from build123d import *

# Parameters (mm, degrees)
BOSS_EXTRUDE1_DEPTH          = 25.4
FILLET1_R                    = 0.79375
M2_5_CLEARANCE_HOLE1_D       = 2.9
M2_5X0_45_TAPPED_HOLE1_D     = 2.05
M2_5X0_45_TAPPED_HOLE1_DEPTH = 3.956117865
M2_5X0_45_TAPPED_HOLE1_TIP   = 0.615882135
F_4_CLEARANCE_HOLE1_D        = 3.2639


with BuildPart() as part:
    # Sketch1 → Boss-Extrude1 (new body)
    with BuildSketch(Plane.XY):
        with BuildLine():
            Line((-4.7625, 2.38125), (4.7625, 2.38125))
            Line((4.7625, 2.38125), (4.7625, 23.01875))
            Line((4.7625, 23.01875), (9.525, 23.01875))
            Line((9.525, 23.01875), (9.525, 5.55625))
            ThreePointArc((9.525, 5.55625), (10.45493597, 3.31118597), (12.7, 2.38125))
            Line((12.7, 2.38125), (22.225, 2.38125))
            Line((22.225, 2.38125), (22.225, -2.38125))
            Line((22.225, -2.38125), (-22.225, -2.38125))
            Line((-22.225, -2.38125), (-22.225, 2.38125))
            Line((-22.225, 2.38125), (-12.7, 2.38125))
            ThreePointArc((-12.7, 2.38125), (-10.45493597, 3.31118597), (-9.525, 5.55625))
            Line((-9.525, 5.55625), (-9.525, 23.01875))
            Line((-9.525, 23.01875), (-4.7625, 23.01875))
            Line((-4.7625, 23.01875), (-4.7625, 2.38125))
        make_face()
    extrude(amount=BOSS_EXTRUDE1_DEPTH)

    # Fillet1
    fillet1_edges = [part.edges().sort_by_distance(p)[0] for p in [
        (-4.7625, 2.38125, 12.7),
        (4.7625, 2.38125, 12.7),
    ]]
    fillet(fillet1_edges, radius=FILLET1_R)

    # M2.5 Clearance Hole1 (through all)
    with Locations(Plane(origin=(0, 2.38125, 0), x_dir=(1, 0, 0), z_dir=(0, 1, 0))):
        with Locations((17.5006, -4.70027), (17.5006, -20.69973), (-17.5006, -20.69973), (-17.5006, -4.70027)):
            Hole(M2_5_CLEARANCE_HOLE1_D / 2)

    # M2.5x0.45 Tapped Hole1
    with Locations(Plane(origin=(0, -2.38125, 0), x_dir=(-1, 0, 0), z_dir=(0, -1, 0))):
        with Locations((-7.78002, -4.70027), (7.78002, -4.70027), (7.78002, -20.69973), (-7.78002, -20.69973)):
            Hole(M2_5X0_45_TAPPED_HOLE1_D / 2, depth=M2_5X0_45_TAPPED_HOLE1_DEPTH)
            with Locations((0, 0, -(M2_5X0_45_TAPPED_HOLE1_DEPTH + M2_5X0_45_TAPPED_HOLE1_TIP / 2))):  # 118° drill point
                Cone(0, M2_5X0_45_TAPPED_HOLE1_D / 2, M2_5X0_45_TAPPED_HOLE1_TIP, mode=Mode.SUBTRACT)

    # #4 Clearance Hole1 (through all)
    with Locations(Plane.ZY.offset(9.525)):
        with Locations((6.35, 18.25625), (19.05, 18.25625), (19.05, 8.73125), (6.35, 8.73125), (12.7, 13.49375)):
            Hole(F_4_CLEARANCE_HOLE1_D / 2)


solid = part.part
Can you work these out from the model? Positions are in its coordinate system, mm. A direction names the side the tool comes from. Round coordinates to 2 decimals unless told otherwise and drop trailing zeros. Loops run counter-clockwise (first coordinate to the right, second up) from the corner with the lowest first, then second, coordinate; pieces in that order, holes last. Notation, with made-up numbers: (85, 72) - (101, 72) arc R15 cw to (101, 99) - close; hole circle Ø11 at (73.5, 18). An arc over 180 degrees is marked (long way). Use CSV: the item, a comma, the result in double quotes. Start each with the question number.
1) For pin 1 Ø3 at (x, z) = (-18.5, 12.5) entering from +Y; pin 2 Ø6 at (y, z) = (14, 15) entering from +X (3 decimals); pin 3 Ø5 at (y, z) = (10.5, 17) entering from -X (3 decimals), each with a flat end and sliding along its axis, tell me the tip position at first contact or that it passes through.
2) If we section it at A-A on z = 12.7: Count the separate pieces of the cut face and the enclosed holes in it, plus the area to 3 significant figures.
3) Please list where these lines run through material, in increasing order: probe 1 along Y at (x, z) = (-7.5, 6.35); probe 2 along X at (y, z) = (20, 19.75) (1 decimal); probe 3 along Z at (x, y) = (-6.5, 18.5). Write a range as [from, to].
4) We'd pull the mould along X, two halves only. Please class faces 1 (the cylindrical face through (8.331, -0.375, 3.836)), 2 (the flat face through (9.525, 16, 13)), 3 (the flat face through (-9.525, 16, 13)), 4 (the cylindrical face through (7.18, 8.8, 20.68)): released by +X, released by -X, zero draft, split by the parting line, or undercut.
5) For faces 5 (the flat face through (0, 2.381, 13)), 6 (the cylindrical face through (8.331, -0.375, 19.835)), 7 (the flat face through (-2, 2, 25.4)), which set-ups out of +Z, -Z, +X, -X, +Y, -Y let a thin tool reach every point of the face, with its end or its side?
6) If we section it at D-D on x = -14: Write out the boundary of the cut face in (y, z), plus the area to 3 significant figures.
7) If we section it at B-B on x = 6: Write out the boundary of the cut face in (y, z).
Geometry results:
1,pin 1,"stops at y = 2.38"
1,pin 2,"stops at x = 9.525"
1,pin 3,"stops at x = -9.525"
2,separate pieces,"3"
2,enclosed holes,"0"
2,area,"382 mm2"
3,probe 1,"y = [-2.38, 7.1], [10.36, 16.62], [19.89, 23.02]"
3,probe 2,"x = [-9.5, -4.8], [4.8, 9.5]"
3,probe 3,"z = [0, 4.74], [7.96, 17.44], [20.66, 25.4]"
4,face 1,"undercut"
4,face 2,"released by +X"
4,face 3,"released by -X"
4,face 4,"zero draft"
5,face 5,"+Z, -Z, +Y"
5,face 6,"-Y"
5,face 7,"+Z, +X, -X, +Y, -Y"
6,outline,"(-2.38, 0) - (2.38, 0) - (2.38, 25.4) - (-2.38, 25.4) - close"
6,area,"121 mm2"
7,outline,"(-2.38, 0) - (23.02, 0) - (23.02, 25.4) - (-2.38, 25.4) - close; hole circle Ø3.26 at (8.73, 6.35); hole circle Ø3.26 at (8.73, 19.05); hole circle Ø3.26 at (13.49, 12.7); hole circle Ø3.26 at (18.26, 6.35); hole circle Ø3.26 at (18.26, 19.05)"
